Verification items for the finished model (mm, model axes). A direction names the side the tool comes from. Coordinates: 2 decimals unless noted, no trailing zeros. Order: outer loops, then holes, each group sorted by start corner. A loop starts at its lowest first (then second) coordinate and runs counter-clockwise, first axis right, second up. Notation, with made-up numbers: (52, 15.5) -> (57, 15.5) arc R30 cw to (57, 41.5) -> close; hole circle Ø11 at (4.25, -25). An arc over 180 degrees is marked (long way). Write item = value, one per line. Start each with the question number.
1. Cross-section at B-B on x = 17. Record the cut outline in (y, z), plus the area to 3 significant figures.
2. Cross-section at C-C on z = 43.5. Record the cut outline in (x, y), plus the area to 3 significant figures.
3. Release check for a two-part mould opening along Z. For faces 3 (the cylindrical face through (26.9, 21.93, 27.86)), 4 (the cylindrical face through (0.33, 21.93, 49.85)), 5 (the cylindrical face through (0.36, 21.93, 54.4)), 6 (the flat face through (0, 2, 49.25)) record: +Z half, -Z half, draft (parallel to the pull), parting line (faces both ways), or undercut.
4. Thickness scan on line 1 along X through (y, z) = (-1.5, 21); line 2 along Z through (x, y) = (14, 6); line 3 along Y through (x, z) = (-9, 12). Record the ranges inside material, lowest first. Write a range as from..to.
5. Set-up check for faces 1 (the cylindrical face through (0.36, 21.93, 0.6)), 2 (the flat face through (0, -17.5, 27)): record each of +Z, -Z, +X, -X, +Y, -Y from which the full face is reachable in a straight line by a thin tool's end or side.
6. Cross-section at A-A on y = 5. Record the cut outline in (x, z).
from build123d import *

# Parameters (mm, degrees)
SKETCH1_W           = 55
SKETCH1_H           = 45
BOSS_EXTRUDE1_DEPTH = 55
SKETCH2_W           = 43.5
SKETCH2_H           = 43.5
CUT_EXTRUDE1_DEPTH  = 40
FILLET2_R           = 2


with BuildPart() as part:
    # Sketch1 → Boss-Extrude1 (new body)
    with BuildSketch(Plane.XY):
        Rectangle(SKETCH1_W, SKETCH1_H)
    extrude(amount=BOSS_EXTRUDE1_DEPTH)

    # Sketch2 → Cut-Extrude1 (cut)
    with BuildSketch(Plane(origin=(0, 22.5, 0), x_dir=(1, 0, 0), z_dir=(0, 1, 0))):
        with Locations((0, -27.5)):
            Rectangle(SKETCH2_W, SKETCH2_H)
    extrude(amount=-CUT_EXTRUDE1_DEPTH, mode=Mode.SUBTRACT)

    # Fillet2
    fillet2_edges = [part.edges().sort_by_distance(p)[0] for p in [
        (-27.5, 0, 55),
        (21.75, 22.5, 27.5),
        (0, 22.5, 5.75),
        (-21.75, 22.5, 27.5),
        (0, 22.5, 49.25),
        (27.5, 0, 55),
        (-27.5, 0, 0),
        (0, 22.5, 0),
        (27.5, 0, 0),
        (0, 22.5, 55),
        (-27.5, 22.5, 27.5),
        (27.5, 22.5, 27.5),
    ]]
    fillet(fillet2_edges, radius=FILLET2_R)


solid = part.part
Worked out:
q1.outline = (-22.5, 0) -> (20.5, 0) arc R2 ccw to (22.5, 2) -> (22.5, 3.75) arc R2 ccw to (20.5, 5.75) -> (-17.5, 5.75) -> (-17.5, 49.25) -> (20.5, 49.25) arc R2 ccw to (22.5, 51.25) -> (22.5, 53) arc R2 ccw to (20.5, 55) -> (-22.5, 55) -> close
q1.area = 732 mm²
q2.outline = (-27.5, -22.5) -> (27.5, -22.5) -> (27.5, 20.5) arc R2 ccw to (25.5, 22.5) -> (23.75, 22.5) arc R2 ccw to (21.75, 20.5) -> (21.75, -17.5) -> (-21.75, -17.5) -> (-21.75, 20.5) arc R2 ccw to (-23.75, 22.5) -> (-25.5, 22.5) arc R2 ccw to (-27.5, 20.5) -> close
q2.area = 732 mm²
q3.face_3 = draft
q3.face_4 = undercut
q3.face_5 = +Z half
q3.face_6 = undercut
q4.line_1 = -27.5..-21.75, 21.75..27.5
q4.line_2 = 0..5.75, 49.25..55
q4.line_3 = -22.5..-17.5
q5.face_1 = -Z, +X, -X, +Y
q5.face_2 = +Y
q6.outline = (-27.5, 2) arc R2 ccw to (-25.5, 0) -> (25.5, 0) arc R2 ccw to (27.5, 2) -> (27.5, 53) arc R2 ccw to (25.5, 55) -> (-25.5, 55) arc R2 ccw to (-27.5, 53) -> close; hole (-21.75, 5.75) -> (21.75, 5.75) -> (21.75, 49.25) -> (-21.75, 49.25) -> close
